Answer from the drawing. Dimensions are ordinates in mm from the lowest x, y and z of the part. A direction names the side the tool comes from. Round coordinates to 2 decimals unless told otherwise and drop trailing zeros. Loops run counter-clockwise (first coordinate to the right, second up) from the corner with the lowest first, then second, coordinate; pieces in that order, holes last. Notation, with made-up numbers: (30.5, -23) - (34.5, -23) arc R5 cw to (34.5, -15) - close; hole circle Ø11 at (-22.75, -25). An arc over 180 degrees is marked (long way). Answer as CSV lines item,"result".
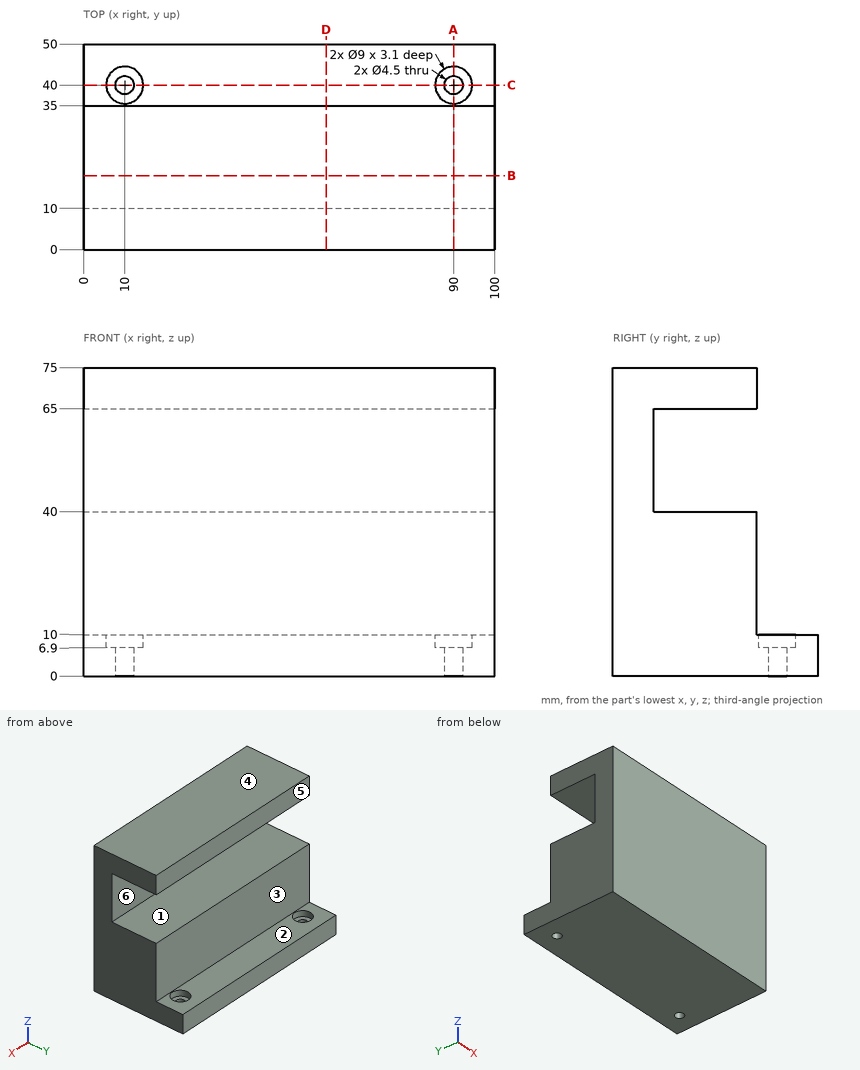
1) A cutting plane is placed at C-C, the plane y = 40. Determine the outline of the cut face in (x, z), plus the area to 3 significant figures.
Entries:
outline,"(0, 0) - (7.75, 0) - (7.75, 6.9) - (5.5, 6.9) - (5.5, 10) - (0, 10) - close; (12.25, 0) - (87.75, 0) - (87.75, 6.9) - (85.5, 6.9) - (85.5, 10) - (14.5, 10) - (14.5, 6.9) - (12.25, 6.9) - close; (92.25, 0) - (100, 0) - (100, 10) - (94.5, 10) - (94.5, 6.9) - (92.25, 6.9) - close"
area,"882 mm^2"
2) The mould has two halves that part along Z. Classify the marked faces 1, 2 and 3: pulls with the +Z half, pulls with the -Z half, needs draft (parallel to the pull), parting line crosses it, or undercut.
Entries:
face 1,"undercut"
face 2,"pulls with the +Z half"
face 3,"needs draft"
3) A cutting plane is placed at B-B, the plane y = 18. Determine the outline of the cut face in (x, z).
Entries:
outline,"(0, 0) - (100, 0) - (100, 40) - (0, 40) - close; (0, 65) - (100, 65) - (100, 75) - (0, 75) - close"
4) A cutting plane is placed at D-D, the plane x = 59. Determine the outline of the cut face in (y, z).
Entries:
outline,"(0, 0) - (50, 0) - (50, 10) - (35, 10) - (35, 40) - (10, 40) - (10, 65) - (35, 65) - (35, 75) - (0, 75) - close"
5) Each of these flat-tipped pins is pushed along its axis until it touches: P1, Ø2.5, axis at x = 91, y = 42, coming from the +Z side; P2, Ø12, axis at x = 56.5, y = 45.5, coming from the +Z side; P3, Ø5, axis at x = 39, z = 69.5, coming from the +Y side. Where does it stop, or does it pass through?
Entries:
P1,"stops at z = 6.9"
P2,"stops at z = 10"
P3,"stops at y = 35"
6) Find the intervals of material crossed by line 1 (Y direction, x = 10, z = 2.5); line 2 (Z direction, x = 61, y = 17); line 3 (Y direction, x = 90, z = 8), in increasing order.
Entries:
line 1,"y = 0 to 37.75, 42.25 to 50"
line 2,"z = 0 to 40, 65 to 75"
line 3,"y = 0 to 35.5, 44.5 to 50"
7) A cutting plane is placed at A-A, the plane x = 90. Determine the outline of the cut face in (y, z), plus the area to 3 significant figures.
Entries:
outline,"(0, 0) - (37.75, 0) - (37.75, 6.9) - (35.5, 6.9) - (35.5, 10) - (35, 10) - (35, 40) - (10, 40) - (10, 65) - (35, 65) - (35, 75) - (0, 75) - close; (42.25, 0) - (50, 0) - (50, 10) - (44.5, 10) - (44.5, 6.9) - (42.25, 6.9) - close"
area,"2,090 mm^2"
8) A tool of negligible diameter and unlimited length cuts with its end or side. For the marked faces 4, 5 and 6, from which of +Z, -Z, +X, -X, +Y, -Y can it reach the whole face along a straight path? Write none if from no direction.
Entries:
face 4,"+Z, +X, -X, +Y, -Y"
face 5,"+Z, +X, -X, +Y"
face 6,"+X, -X, +Y"
